Autodesk Inventor part; units mm, degrees
ref_plane "YZ Plane" through (0, 0, 0) normal (1, 0, 0) x (0, 1, 0)
ref_plane "XZ Plane" through (0, 0, 0) normal (0, 1, 0) x (-1, 0, 0)
ref_plane "XY Plane" through (0, 0, 0) normal (0, 0, 1) x (1, 0, 0)
sketch "Sketch6" plane through (0, 0, 0) normal (0, 0, 1) x (1, 0, 0)
  line L0 (0, 0) -> (43, 24.8261)
  line L1 (0, 0) -> (-43, 24.8261)
  line L2 (0, 0) -> (0, 440) construction
  line L3 (-43, 24.8261) -> (43, 24.8261) construction
  line L4 (43, 24.8261) -> (43, 460)
  line L5 (43, 460) -> (-43, 460)
  line L6 (-43, 460) -> (-43, 24.8261)
  circle A0 centre (0, 440) radius 8.5
  circle A1 centre (0, 0) radius 440 construction
  circle A2 centre (0, 0) radius 460 construction
  dimension "d44" = 880
  dimension "d40" = 120
  dimension "d42" = 86
  dimension "d43" = 17
  dimension "d45" = 920
extrude "Plate3" add sketch "Sketch6" along normal blind 3
equation "\"d46\" = Thickness"
equation "\"BendReliefWidth\" = Thickness"
equation "\"BendReliefDepth\" = 0.5 * Thickness"
equation "\"CornerReliefSize\" = 4 * Thickness"
equation "\"MinimumRemnant\" = 2 * Thickness"
equation "\"TransitionRadius\" = BendRadius"
equation "\"JacobiRadiusSize\" = BendRadius"
equation "\"GapSize\" = Thickness"
properties part number "PRS 940-96 leg floor pattern" material "Stainless Steel"
For this review, take the finished solid that the model builds, in its own axes (mm). Coordinates: 2 decimals unless noted, no trailing zeros. Loops run counter-clockwise (first coordinate to the right, second up) from the corner with the lowest first, then second, coordinate; pieces in that order, holes last. Notation, with made-up numbers: (38, 0) - (53, 0) arc R30 ccw to (53, 37) - close; hole circle Ø9 at (44, 36.5). An arc over 180 degrees is marked (long way). Return JSON: item names as keys, results as strings.
Item 1: Take a section at C-C (x = 26). Give the boundary of the cut face in (y, z).
Determined:
{"outline": "(15.01, 0) - (460, 0) - (460, 3) - (15.01, 3) - close"}
Item 2: Take a section at B-B (z = 0.8). Give the boundary of the cut face in (x, y).
Determined:
{"outline": "(-43, 24.83) - (0, 0) - (43, 24.83) - (43, 460) - (-43, 460) - close; hole circle Ø17 at (0, 440)"}
Item 3: Insertion check: pin 1 (2 mm diameter, centred on x = -30, y = 109, fed in from -Z); pin 2 (1.5 mm diameter, centred on x = -18, z = 2, fed in from -Y). Each pin has a flat end and moves straight along its axis. Give the tip position at first contact, or say it passes through.
Determined:
{"pin 1": "stops at z = 0", "pin 2": "stops at y = 9.96"}
Item 4: For line 1 (Y direction, x = 0, z = 1.95); line 2 (Y direction, x = 7.5, z = 0.2); line 3 (Y direction, x = 37.5, z = 2.65), list the stretches that pass through material, from the lowest coordinate up.
Determined:
{"line 1": "y = 0 to 431.5, 448.5 to 460", "line 2": "y = 4.33 to 436, 444 to 460", "line 3": "y = 21.65 to 460"}
Item 5: Take a section at D-D (x = -13.5). Give the boundary of the cut face in (y, z).
Determined:
{"outline": "(7.79, 0) - (460, 0) - (460, 3) - (7.79, 3) - close"}
Item 6: Mouldability with a two-part tool opening along Y and no side actions: class faces 1 (the cylindrical face through (-1.107, 431.572, 1.479)), 2 (the flat face through (-1, 233, 3)), 3 (the flat face through (21.2, 12.24, 1.48)) as pulls with the +Y half, pulls with the -Y half, needs draft (parallel to the pull), parting line crosses it, or undercut.
Determined:
{"face 1": "undercut", "face 2": "needs draft", "face 3": "pulls with the -Y half"}
Item 7: Take a section at A-A (y = 440). Give the boundary of the cut face in (x, z).
Determined:
{"outline": "(-43, 0) - (-8.5, 0) - (-8.5, 3) - (-43, 3) - close; (8.5, 0) - (43, 0) - (43, 3) - (8.5, 3) - close"}
